Check sheet for the modelled part. Datum: model origin and axes. Units: mm. A direction names the side the tool comes from. Give positions to 0.01 mm unless a question says otherwise; leave off trailing zeros. Order: outer loops, then holes, each group sorted by start corner. A loop starts at its lowest first (then second) coordinate and runs counter-clockwise, first axis right, second up.
Item 1: Material ranges on line 1 along Y through (x, z) = (0, 7.75) (3 decimals); line 2 along X through (y, z) = (47, 2); line 3 along Y through (x, z) = (-12, 4.25), recorded low to high.
Item 2: Access from +Z, -Z, +X, -X, +Y, -Y to the whole of each face (thin tool, end or side, straight path). Record for faces 4 (the cylindrical face through (0.56, -53.97, 9.39)), 5 (the flat face through (-29, -28.575, 9)), 6 (the flat face through (29, -28.575, 9)).
Item 3: Sectioned sample at D-D on x = -15.5. Record the boundary of the cut face in (y, z).
Item 4: Gauge pin test, flat ends, axial feed: P1, Ø1.5, axis at x = 1.5, z = 3, coming from the -Y side; P2, Ø1.9, axis at x = 29, z = 10.5, coming from the -Y side (3 decimals); P3, Ø5, axis at x = 9.5, z = 11, coming from the -Y side. Record the tip position at first contact, or that the pin passes through.
Item 5: Sectioned sample at B-B on z = 11.75. Record the boundary of the cut face in (x, y) (3 decimals).
Item 6: Release check for a two-part mould opening along Y. For faces 1 (the cylindrical face through (-0.698, 60.317, 9.392)), 2 (the flat face through (0, 4, 0)), 3 (the cylindrical face through (-0.413, -25.427, 9.658)) record: released by +Y, released by -Y, zero draft, split by the parting line, or undercut.
Item 7: Sectioned sample at C-C on y = -34.5. Record the boundary of the cut face in (x, z), and give its area (3 significant figures).
Item 8: Sectioned sample at A-A on x = 0. Record the boundary of the cut face in (y, z) (3 decimals), and give its area (3 significant figures).
from build123d import *

# Parameters (mm, degrees)
BOSS_EXTRUDE1_DEPTH         = 19.05
F_1_4_0_25_DIAMETER_HOLE1_D = 6.35


with BuildPart() as part:
    # Sketch2 → Boss-Extrude1 (new body)
    with BuildSketch(Plane.XY):
        with BuildLine():
            Line((31.75, 28.575), (31.75, -28.575))
            Line((31.75, -28.575), (25.4, -28.575))
            ThreePointArc((25.4, -28.575), (0, -53.975), (-25.4, -28.575))
            Line((-25.4, -28.575), (-31.75, -28.575))
            Line((-31.75, -28.575), (-31.75, 28.575))
            ThreePointArc((-31.75, 28.575), (0, 60.325), (31.75, 28.575))
        make_face()
    extrude(amount=BOSS_EXTRUDE1_DEPTH)

    # 1/4 (0.25) Diameter Hole1 (through all)
    with Locations(Plane(origin=(0, 0, 0), x_dir=(-1, 0, 0), z_dir=(0, 0, -1))):
        with Locations((0, -28.575)):
            Hole(F_1_4_0_25_DIAMETER_HOLE1_D / 2)


solid = part.part
Report:
1. line 1: y = -53.975 to -31.75, -25.4 to 60.325
1. line 2: x = -25.86 to 25.86
1. line 3: y = -50.96 to 57.97
2. face 4: +Z, -Z, -Y
2. face 5: +Z, -Z, -X, -Y
2. face 6: +Z, -Z, +X, -Y
3. outline: (-48.7, 0) - (56.28, 0) - (56.28, 19.05) - (-48.7, 19.05) - close
4. P1: stops at y = -53.96
4. P2: stops at y = -28.575
4. P3: stops at y = -52.99
5. outline: (-31.75, -28.575) - (-25.4, -28.575) arc R25.4 ccw to (25.4, -28.575) - (31.75, -28.575) - (31.75, 28.575) arc R31.75 ccw to (-31.75, 28.575) - close; hole circle Ø6.35 at (0, -28.575)
6. face 1: released by +Y
6. face 2: zero draft
6. face 3: undercut
7. outline: (-24.7, 0) - (24.7, 0) - (24.7, 19.05) - (-24.7, 19.05) - close
7. area: 941 mm2
8. outline: (-53.975, 0) - (-31.75, 0) - (-31.75, 19.05) - (-53.975, 19.05) - close; (-25.4, 0) - (60.325, 0) - (60.325, 19.05) - (-25.4, 19.05) - close
8. area: 2,060 mm2
